Can you work these out from the model? Positions are in its coordinate system, mm. Round coordinates to 2 decimals unless told otherwise and drop trailing zeros. Order: outer loops, then holes, each group sorted by start corner. A loop starts at its lowest first (then second) coordinate and runs counter-clockwise, first axis right, second up. Notation, with made-up numbers: (47, 42.5) -> (66, 42.5) arc R16 cw to (66, 62.5) -> close; hole circle Ø7 at (74, 56.25). An arc over 180 degrees is marked (long way). One line per item, written item: value.
```python
from build123d import *

# Parameters (mm, degrees)
BOSS_EXTRUDE1_DEPTH = 1.9
SKETCH2_R           = 0.225
BOSS_EXTRUDE2_DEPTH = 31.5


with BuildPart() as part:
    # Sketch1 → Boss-Extrude1 (new body)
    with BuildSketch(Plane(origin=(0, 0, 0), x_dir=(1, 0, 0), z_dir=(0, 1, 0))):
        with BuildLine():
            Line((-2.8, 2.298937026), (-2.8, 0))
            Line((-2.8, 0), (2.8, 0))
            Line((2.8, 0), (2.8, 2.298937026))
            ThreePointArc((2.8, 2.298937026), (1.49982595, 3.096723441), (0, 3.375))
            ThreePointArc((0, 3.375), (-1.49982595, 3.096723441), (-2.8, 2.298937026))
        make_face()
    boss_extrude1 = extrude(amount=BOSS_EXTRUDE1_DEPTH)

    # Sketch2 → Boss-Extrude2 (add)
    with BuildSketch(Plane.XZ):
        with Locations(Location((0, -2.15, 0), (0, 0, 90))):
            Circle(SKETCH2_R)
    boss_extrude2 = extrude(amount=BOSS_EXTRUDE2_DEPTH)

    # Mirror2: Boss-Extrude1, Boss-Extrude2 across plane
    add(boss_extrude1.mirror(Plane.XY))
    add(boss_extrude2.mirror(Plane.XY))


solid = part.part
```
Q1. Will these pins go through, and if not, where does the flat tip stop? pin 1 Ø1.5 at (x, y) = (1.5, -7) entering from -Z; pin 2 Ø2 at (x, y) = (-1, -2.5) entering from -Z (3 decimals); pin 3 Ø1.5 at (y, z) = (-13.5, 2.5) entering from -X (3 decimals).
Answers below:
pin 1: through
pin 2: z = -2.375
pin 3: x = -0.225
Q2. Please list where these lines run through material, in increasing order: line 1 along Y through (x, z) = (0.1, 2.5); line 2 along X through (y, z) = (-17.5, 2).
Answers below:
line 1: 0 to 1.9
line 2: -0.17 to 0.17
Q3. I want a section at C-C on x = 1.3. List the corners of the cut face in (y, z) for me.
Answers below:
outline: (0, -3.17) -> (1.9, -3.17) -> (1.9, 3.17) -> (0, 3.17) -> close
Q4. I want a section at B-B on z = -0.75. List the corners of the cut face in (x, y) for me.
Answers below:
outline: (-2.8, 0) -> (2.8, 0) -> (2.8, 1.9) -> (-2.8, 1.9) -> close
Q5. I want a section at A-A on y = -14. List the corners of the cut face in (x, z) for me (3 decimals).
Answers below:
outline: circle Ø0.45 at (0, -2.15); circle Ø0.45 at (0, 2.15)
